Check sheet for the drawn part. Datum: minimum x, y, z corner. Units: mm. Round coordinates to 2 decimals unless told otherwise and drop trailing zeros. Write each loop counter-clockwise with the first axis right and the second up, starting at its lowest first coordinate (ties: lowest second). Pieces come first, ordered by that corner, then holes.
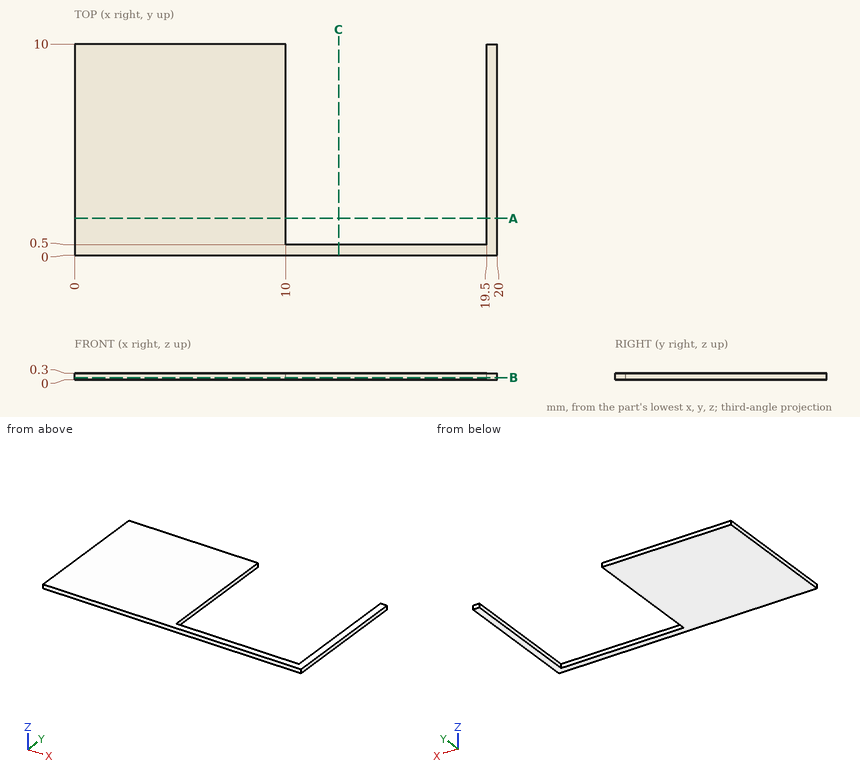
Q1. Material ranges on line 1 along X through (y, z) = (5.25, 0.15); line 2 along Y through (x, z) = (10.25, 0.2), recorded low to high.
Recorded:
line 1: x = 0 to 10, 19.5 to 20
line 2: y = 0 to 0.5
Q2. Sectioned sample at C-C (x = 12.5). Enter the section's corners in (y, z).
Recorded:
outline: (0, 0) - (0.5, 0) - (0.5, 0.3) - (0, 0.3) - close
Q3. Sectioned sample at B-B (z = 0.1). Enter the section's corners in (x, y).
Recorded:
outline: (0, 0) - (20, 0) - (20, 10) - (19.5, 10) - (19.5, 0.5) - (10, 0.5) - (10, 10) - (0, 10) - close
Q4. Sectioned sample at A-A (y = 1.75). Enter the section's corners in (x, z), plus the area to 3 significant figures.
Recorded:
outline: (0, 0) - (10, 0) - (10, 0.3) - (0, 0.3) - close; (19.5, 0) - (20, 0) - (20, 0.3) - (19.5, 0.3) - close
area: 3.15 mm2
